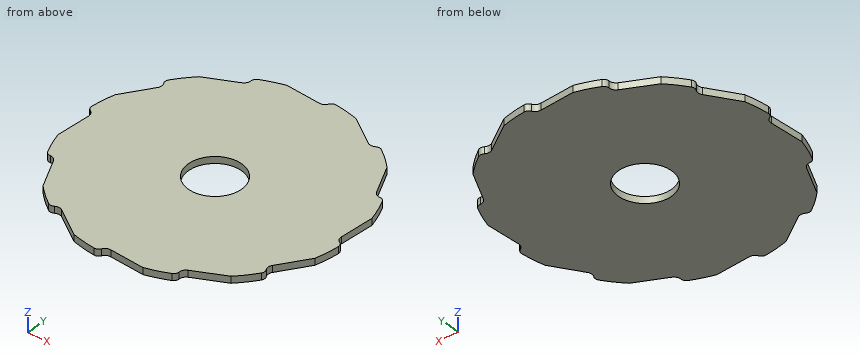
```python
from build123d import *

# Parameters (mm, degrees)
F0_R     = 127
F0_R_2   = 25.4
F1_DEPTH = 6.35
F3_DEPTH = 6.351
F4_R     = 5.08


with BuildPart() as f1:
    # F0 (on Top) → F1 (new body)
    with BuildSketch(Plane.XY):
        Circle(F0_R)
        Circle(F0_R_2, mode=Mode.SUBTRACT)
    extrude(amount=F1_DEPTH)

    # F2 (on face) → F3 (cut, through all)
    with BuildSketch(Plane.XY.offset(6.35)):
        with BuildLine():
            ThreePointArc((-0.4417075975, 120.4113812744), (4.3658298911, 122.1349231885), (6.349286539, 126.8411863727))
            ThreePointArc((6.349286539, 126.8411863727), (-13.4231750663, 126.288631203), (-32.870018728, 122.6725799387))
            Line((-32.870018728, 122.6725799387), (-0.4417075975, 120.4113812744))
        make_face()
        with BuildLine():
            ThreePointArc((-60.5882206377, 104.0584612897), (-57.286542, 107.954861116), (-57.9219497477, 113.0223329145))
            ThreePointArc((-57.9219497477, 113.0223329145), (-74.7691262084, 102.6575752978), (-89.8025612107, 89.8025612107))
            Line((-89.8025612107, 89.8025612107), (-60.5882206377, 104.0584612897))
        make_face()
        with BuildLine():
            ThreePointArc((-104.5001688872, 59.8231606367), (-103.5890312249, 64.8483811885), (-106.6730463754, 68.9192366251))
            ThreePointArc((-106.6730463754, 68.9192366251), (-116.0807503642, 51.5195049947), (-122.6725799387, 32.870018728))
            Line((-122.6725799387, 32.870018728), (-104.5001688872, 59.8231606367))
        make_face()
        with BuildLine():
            ThreePointArc((-120.4113812744, -0.4417075975), (-122.1349231885, 4.3658298911), (-126.8411863727, 6.349286539))
            ThreePointArc((-126.8411863727, 6.349286539), (-126.288631203, -13.4231750663), (-122.6725799387, -32.870018728))
            Line((-122.6725799387, -32.870018728), (-120.4113812744, -0.4417075975))
        make_face()
        with BuildLine():
            ThreePointArc((-104.0584612897, -60.5882206377), (-107.954861116, -57.286542), (-113.0223329145, -57.9219497477))
            ThreePointArc((-113.0223329145, -57.9219497477), (-102.6575752978, -74.7691262084), (-89.8025612107, -89.8025612107))
            Line((-89.8025612107, -89.8025612107), (-104.0584612897, -60.5882206377))
        make_face()
        with BuildLine():
            ThreePointArc((-59.8231606367, -104.5001688872), (-64.8483811885, -103.5890312249), (-68.9192366251, -106.6730463754))
            ThreePointArc((-68.9192366251, -106.6730463754), (-51.5195049947, -116.0807503642), (-32.870018728, -122.6725799387))
            Line((-32.870018728, -122.6725799387), (-59.8231606367, -104.5001688872))
        make_face()
        with BuildLine():
            ThreePointArc((0.4417075975, -120.4113812744), (-4.3658298911, -122.1349231885), (-6.349286539, -126.8411863727))
            ThreePointArc((-6.349286539, -126.8411863727), (13.4231750663, -126.288631203), (32.870018728, -122.6725799387))
            Line((32.870018728, -122.6725799387), (0.4417075975, -120.4113812744))
        make_face()
        with BuildLine():
            ThreePointArc((60.5882206377, -104.0584612897), (57.286542, -107.954861116), (57.9219497477, -113.0223329145))
            ThreePointArc((57.9219497477, -113.0223329145), (74.7691262084, -102.6575752978), (89.8025612107, -89.8025612107))
            Line((89.8025612107, -89.8025612107), (60.5882206377, -104.0584612897))
        make_face()
        with BuildLine():
            ThreePointArc((104.5001688872, -59.8231606367), (103.5890312249, -64.8483811885), (106.6730463754, -68.9192366251))
            ThreePointArc((106.6730463754, -68.9192366251), (116.0807503642, -51.5195049947), (122.6725799387, -32.870018728))
            Line((122.6725799387, -32.870018728), (104.5001688872, -59.8231606367))
        make_face()
        with BuildLine():
            ThreePointArc((120.4113812744, 0.4417075975), (122.1349231885, -4.3658298911), (126.8411863727, -6.349286539))
            ThreePointArc((126.8411863727, -6.349286539), (126.288631203, 13.4231750663), (122.6725799387, 32.870018728))
            Line((122.6725799387, 32.870018728), (120.4113812744, 0.4417075975))
        make_face()
        with BuildLine():
            ThreePointArc((104.0584612897, 60.5882206377), (107.954861116, 57.286542), (113.0223329145, 57.9219497477))
            ThreePointArc((113.0223329145, 57.9219497477), (102.6575752978, 74.7691262084), (89.8025612107, 89.8025612107))
            Line((89.8025612107, 89.8025612107), (104.0584612897, 60.5882206377))
        make_face()
        with BuildLine():
            ThreePointArc((59.8231606367, 104.5001688872), (64.8483811885, 103.5890312249), (68.9192366251, 106.6730463754))
            ThreePointArc((68.9192366251, 106.6730463754), (51.5195049947, 116.0807503642), (32.870018728, 122.6725799387))
            Line((32.870018728, 122.6725799387), (59.8231606367, 104.5001688872))
        make_face()
    extrude(amount=-F3_DEPTH, mode=Mode.SUBTRACT)

    # F4
    f4_edges = [f1.edges().sort_by_distance(p)[0] for p in [
        (6.349287, 126.841186, 3.175),
        (68.919237, 106.673046, 3.175),
        (113.022333, 57.92195, 3.175),
        (126.841186, -6.349287, 3.175),
        (106.673046, -68.919237, 3.175),
        (-57.92195, 113.022333, 3.175),
        (-106.673046, 68.919237, 3.175),
        (-126.841186, 6.349287, 3.175),
        (-113.022333, -57.92195, 3.175),
        (-68.919237, -106.673046, 3.175),
        (-6.349287, -126.841186, 3.175),
        (57.92195, -113.022333, 3.175),
    ]]
    fillet(f4_edges, radius=F4_R)


solid = f1.part
```
The listing builds one solid part. Answer for the finished solid, in the listing's coordinates (mm). Round coordinates to 2 decimals unless told otherwise and drop trailing zeros. Write each loop counter-clockwise with the first axis right and the second up, starting at its lowest first coordinate (ties: lowest second). Pieces come first, ordered by that corner, then holes. Notation, with made-up numbers: (-6, -16) -> (23, -16) arc R18 cw to (23, 14) -> close; hole circle Ø5 at (55.5, 52.25). An arc over 180 degrees is marked (long way). Answer as a JSON object with one key per item and string values. Group by question number.
Q1. Section A-A (x = 20.5) is taken. Write down the section's boundary in (y, z), plus the area to 3 significant figures.
Q2. Section C-C (x = -39) is taken. Write down the section's boundary in (y, z), plus the area to 3 significant figures.
Q3. Each of these flat-tipped pins is pushed along its axis until it touches: pin 1 Ø2 at (y, z) = (-80, 5) entering from +X; pin 2 Ø1 at (x, z) = (49, 1.5) entering from +Y; pin 3 Ø1.5 at (x, z) = (-36.5, 5) entering from +Y. Where does it stop, or does it pass through?
Q4. Section B-B (y = 17) is taken. Write down the section's boundary in (x, z).
Q5. Straight lines are drawn through the part: line 1 along Y through (x, z) = (0, 1.5); line 2 along Y through (x, z) = (-11, 1.25); line 3 along Y through (x, z) = (-39.5, 3.75). For each, find the intervals that lie inside material, in ascending order.
Check values:
{
 "1": {"outline": "(-121.81, 0) -> (-15, 0) -> (-15, 6.35) -> (-121.81, 6.35) -> close; (15, 0) -> (125.33, 0) -> (125.33, 6.35) -> (15, 6.35) -> close", "area": "1,380 mm^2"},
 "2": {"outline": "(-118.54, 0) -> (120.86, 0) -> (120.86, 6.35) -> (-118.54, 6.35) -> close", "area": "1,520 mm^2"},
 "3": {"pin 1": "x = 99.44", "pin 2": "y = 112.13", "pin 3": "y = 121.86"},
 "4": {"outline": "(-125.86, 0) -> (-18.87, 0) -> (-18.87, 6.35) -> (-125.86, 6.35) -> close; (18.87, 0) -> (121.57, 0) -> (121.57, 6.35) -> (18.87, 6.35) -> close"},
 "5": {"line 1": "-120.4 to -25.4, 25.4 to 120.4", "line 2": "-126.52 to -22.89, 22.89 to 121.15", "line 3": "-118.2 to 120.7"}
}
